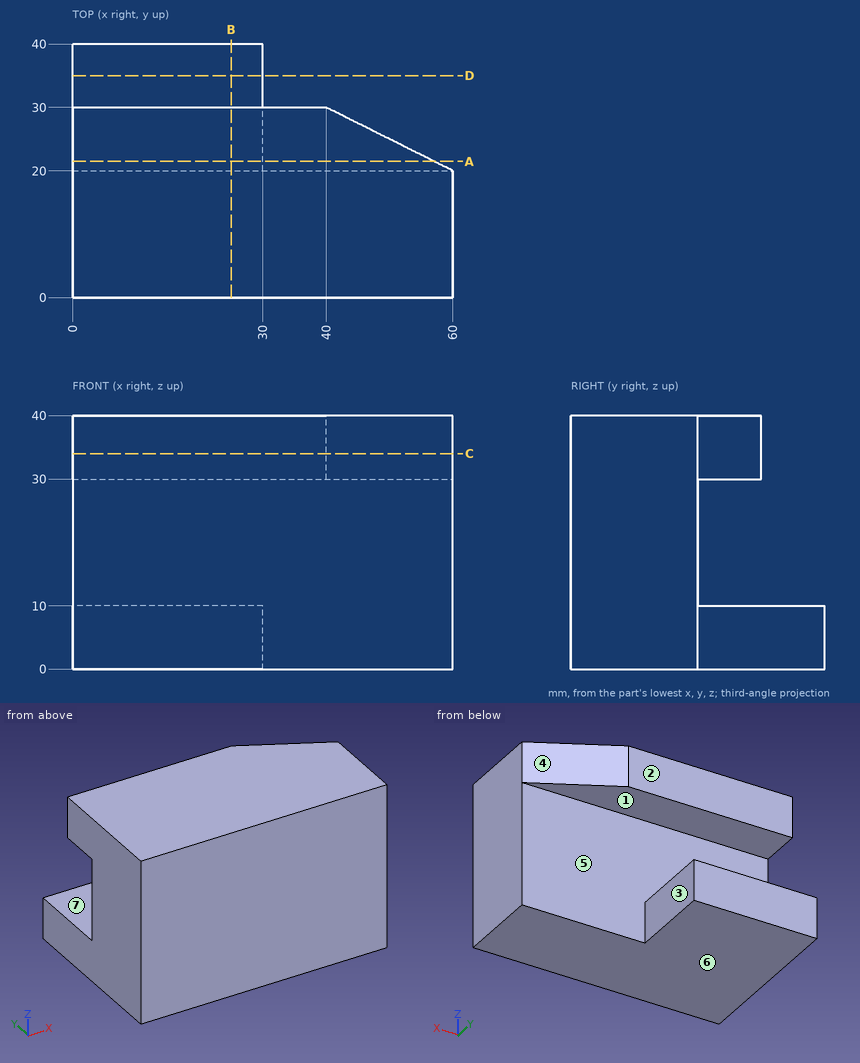
Print and shaded views of the part. All mm, measured from the part's lowest x, y and z. A direction names the side the tool comes from. Coordinates: 2 decimals unless noted, no trailing zeros. Loops run counter-clockwise (first coordinate to the right, second up) from the corner with the lowest first, then second, coordinate; pieces in that order, holes last. Notation, with made-up numbers: (26.25, 77) -> (75.25, 77) arc R19 ccw to (75.25, 111) -> close; hole circle Ø9 at (21, 32.5). An arc over 180 degrees is marked (long way). Use a Markdown table: item, result. Add a question column.
Item 1: Band-saw the part on A-A on y = 21.5. Write the cut outline in (x, z), plus the area to 3 significant figures.
Item 2: Pull direction Z, two halves, no side cores. Call the marked faces 4, 5, 6 and 7: +Z half, -Z half, draft (parallel to the pull), parting line (faces both ways), or undercut.
Item 3: Band-saw the part on D-D on y = 35. Write the cut outline in (x, z), plus the area to 3 significant figures.
Item 4: Band-saw the part on B-B on x = 25. Write the cut outline in (y, z), plus the area to 3 significant figures.
Item 5: Band-saw the part on C-C on z = 34. Write the cut outline in (x, y).
Item 6: Probe probe 1 along Z at (x, y) = (29, 24.5); probe 2 along Y at (x, z) = (36, 24.5); probe 3 along Z at (x, y) = (10, 35). List the from-to ranges inside material, lowest first.
Item 7: Which spindle directions (+Z, -Z, +X, -X, +Y, -Y) get a long thin tool onto all of the face, cutting with end or side? Do the marked faces 1, 2 and 3. Say none if no direction does.
Item 8: Flat gauge pins, fed straight in: P1, Ø11, axis at x = 15, z = 33.5, coming from the +Y side; P2, Ø4, axis at x = 27, z = 21.5, coming from the +Y side; P3, Ø3, axis at y = 30.5, z = 7.5, coming from the +X side; P4, Ø12, axis at y = 31.5, z = 16.5, coming from the -X side. Where does each tip first touch, or does it go through?
Geometry says:
| question | item | result |
|---|---|---|
| 1 | outline | (0, 0) -> (30, 0) -> (30, 10) -> (0, 10) -> close; (0, 30) -> (57, 30) -> (57, 40) -> (0, 40) -> close |
| 1 | area | 870 mm² |
| 2 | face 4 | draft |
| 2 | face 5 | undercut |
| 2 | face 6 | -Z half |
| 2 | face 7 | undercut |
| 3 | outline | (0, 0) -> (30, 0) -> (30, 10) -> (0, 10) -> close |
| 3 | area | 300 mm² |
| 4 | outline | (0, 0) -> (40, 0) -> (40, 10) -> (20, 10) -> (20, 30) -> (30, 30) -> (30, 40) -> (0, 40) -> close |
| 4 | area | 1,100 mm² |
| 5 | outline | (0, 0) -> (60, 0) -> (60, 20) -> (40, 30) -> (0, 30) -> close |
| 6 | probe 1 | 0 to 10, 30 to 40 |
| 6 | probe 2 | 0 to 20 |
| 6 | probe 3 | 0 to 10 |
| 7 | face 1 | +X, -X, +Y |
| 7 | face 2 | +Z, +X, -X, +Y |
| 7 | face 3 | -Z, +X, +Y |
| 8 | P1 | y = 30 |
| 8 | P2 | y = 20 |
| 8 | P3 | x = 30 |
| 8 | P4 | through |
